from build123d import *

# Parameters (mm, degrees)
SKETCH1_W           = 10
SKETCH1_H           = 3
BOSS_EXTRUDE1_DEPTH = 3


with BuildPart() as part:
    # Sketch1 → Boss-Extrude1 (new body)
    with BuildSketch(Plane(origin=(0, 0, 0), x_dir=(0, 0, -1), z_dir=(1, 0, 0))):
        with BuildLine():
            Line((-100, -44), (-100, -60))
            Line((-100, -60), (-80, -60))
            Line((-80, -60), (-80, -50))
            Line((-80, -50), (80, -50))
            Line((80, -50), (80, -60))
            Line((80, -60), (100, -60))
            Line((100, -60), (100, -44))
            Line((100, -44), (97, -44))
            Line((97, -44), (97, -34))
            Line((97, -34), (100, -34))
            Line((100, -34), (100, -24))
            Line((100, -24), (97, -24))
            Line((97, -24), (97, -14))
            Line((97, -14), (100, -14))
            Line((100, -14), (100, -4))
            Line((100, -4), (97, -4))
            Line((97, -4), (97, 6))
            Line((97, 6), (100, 6))
            Line((100, 6), (100, 16))
            Line((100, 16), (97, 16))
            Line((97, 16), (97, 26))
            Line((97, 26), (100, 26))
            Line((100, 26), (100, 36))
            Line((100, 36), (97, 36))
            Line((97, 36), (97, 46))
            Line((97, 46), (100, 46))
            Line((100, 46), (100, 60))
            Line((100, 60), (75.851854343, 53.529523872))
            Line((75.851854343, 53.529523872), (76.628311478, 50.631746394))
            Line((76.628311478, 50.631746394), (66.969053215, 48.043555943))
            Line((66.969053215, 48.043555943), (66.19259608, 50.941333421))
            Line((66.19259608, 50.941333421), (56.533337817, 48.35314297))
            Line((56.533337817, 48.35314297), (57.309794952, 45.455365492))
            Line((57.309794952, 45.455365492), (47.650536689, 42.86717504))
            Line((47.650536689, 42.86717504), (46.874079554, 45.764952519))
            Line((46.874079554, 45.764952519), (37.214821291, 43.176762068))
            Line((37.214821291, 43.176762068), (37.991278427, 40.278984589))
            Line((37.991278427, 40.278984589), (28.332020164, 37.690794138))
            Line((28.332020164, 37.690794138), (27.555563028, 40.588571617))
            Line((27.555563028, 40.588571617), (17.896304765, 38.000381166))
            Line((17.896304765, 38.000381166), (18.672761901, 35.102603687))
            Line((18.672761901, 35.102603687), (9.013503638, 32.514413236))
            Line((9.013503638, 32.514413236), (8.237046503, 35.412190715))
            Line((8.237046503, 35.412190715), (-1.42221176, 32.824000264))
            Line((-1.42221176, 32.824000264), (-0.645754625, 29.926222785))
            Line((-0.645754625, 29.926222785), (-10.305012888, 27.338032334))
            Line((-10.305012888, 27.338032334), (-11.081470023, 30.235809813))
            Line((-11.081470023, 30.235809813), (-20.740728286, 27.647619362))
            Line((-20.740728286, 27.647619362), (-19.964271151, 24.749841883))
            Line((-19.964271151, 24.749841883), (-29.623529414, 22.161651432))
            Line((-29.623529414, 22.161651432), (-30.399986549, 25.059428911))
            Line((-30.399986549, 25.059428911), (-40.059244812, 22.47123846))
            Line((-40.059244812, 22.47123846), (-39.282787677, 19.573460981))
            Line((-39.282787677, 19.573460981), (-48.942045939, 16.98527053))
            Line((-48.942045939, 16.98527053), (-49.718503075, 19.883048009))
            Line((-49.718503075, 19.883048009), (-68.302221487, 14.903555668))
            ThreePointArc((-68.302221487, 14.903555668), (-91.366544651, -0.636913735), (-100, -27.074247963))
            Line((-100, -27.074247963), (-100, -34))
            Line((-100, -34), (-97, -34))
            Line((-97, -34), (-97, -44))
            Line((-97, -44), (-100, -44))
        make_face()
        with Locations((-82, -45.5)):
            Rectangle(SKETCH1_W, SKETCH1_H, mode=Mode.SUBTRACT)
        with Locations((-62, -45.5)):
            Rectangle(SKETCH1_W, SKETCH1_H, mode=Mode.SUBTRACT)
        with Locations((-42, -45.5)):
            Rectangle(SKETCH1_W, SKETCH1_H, mode=Mode.SUBTRACT)
        with Locations((-22, -45.5)):
            Rectangle(SKETCH1_W, SKETCH1_H, mode=Mode.SUBTRACT)
        with Locations((-2, -45.5)):
            Rectangle(SKETCH1_W, SKETCH1_H, mode=Mode.SUBTRACT)
        with Locations((18, -45.5)):
            Rectangle(SKETCH1_W, SKETCH1_H, mode=Mode.SUBTRACT)
        with Locations((38, -45.5)):
            Rectangle(SKETCH1_W, SKETCH1_H, mode=Mode.SUBTRACT)
        with Locations((58, -45.5)):
            Rectangle(SKETCH1_W, SKETCH1_H, mode=Mode.SUBTRACT)
        with Locations((78, -45.5)):
            Rectangle(SKETCH1_W, SKETCH1_H, mode=Mode.SUBTRACT)
    extrude(amount=BOSS_EXTRUDE1_DEPTH)


solid = part.part
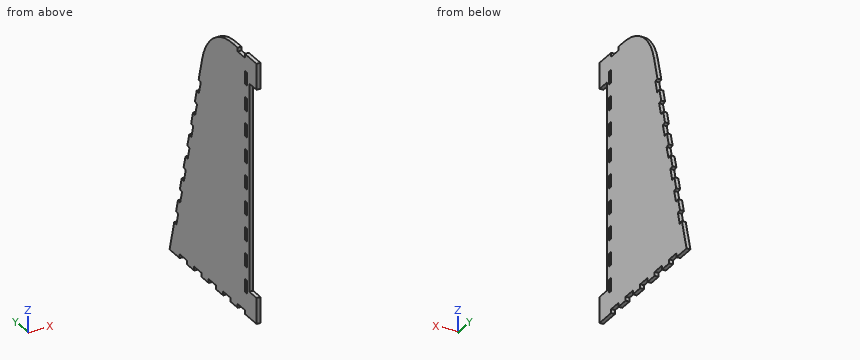
Geometry: final body of the model. Coordinates: model frame, mm. Give positions to 0.01 mm unless a question says otherwise; leave off trailing zeros. Write each loop counter-clockwise with the first axis right and the second up, starting at its lowest first coordinate (ties: lowest second). Pieces come first, ordered by that corner, then holes. Notation, with made-up numbers: M 75,53.25 L 119,53.25 A33 ccw 119,91.25 Z; hole C -34,-11.75 d2. An arc over 180 degrees is marked long. Answer in a Markdown table with one row per item. Add a question column.
(1) Section B-B on x = 2.4. State how many separate pieces and enclosed holes the cut face has, and give its area (3 significant figures).
(2) Section A-A on z = 4. Return loops of the section in (x, y), and give its area (3 significant figures).
(3) Section C-C on y = 11. Return loops of the section in (x, z).
(4) Section D-D on y = -16.5. Return loops of the section in (x, z).
(5) First-contact query: pin 1 (1.5 mm diameter, centred on x = 2, y = -19.5, fed in from -Z); pin 2 (1 mm diameter, centred on x = 1.5, y = 32, fed in from +Z); pin 3 (0.9 mm diameter, centred on x = 1.5, y = -45, fed in from +Z). Flat tips, straight axial feed; report the tip coordinate or a pass-through.
(6) Ray query, line 1 (Y direction, x = 0.65, z = -59.5); line 2 (Y direction, x = 1.8, z = -74); line 3 (Z direction, x = 2.4, y = -48.5). Return the intervals inside material, ascending.
Result set:
| question | item | result |
|---|---|---|
| 1 | separate pieces | 1 |
| 1 | enclosed holes | 9 |
| 1 | area | 16,200 mm^2 |
| 2 | outline | M 0,-50 L 3,-50 L 3,-47 L 0,-47 Z; M 0,-44 L 3,-44 L 3,29.03 L 0,29.03 Z |
| 2 | area | 228 mm^2 |
| 3 | outline | M 0,-100 L 3,-100 L 3,77.97 L 0,77.97 Z |
| 4 | outline | M 0,-97 L 3,-97 L 3,98.84 L 0,98.84 Z |
| 5 | pin 1 | stops at z = -97 |
| 5 | pin 2 | stops at z = 1.34 |
| 5 | pin 3 | stops at z = 100 |
| 6 | line 1 | y = -50 to -47, -44 to 49.15 |
| 6 | line 2 | y = -50 to -47, -44 to 49.93 |
| 6 | line 3 | z = -100 to 100 |
